Geometry check sheet. Reference: the model listing, model coordinates, mm. A direction names the side the tool comes from. Round coordinates to 2 decimals unless told otherwise and drop trailing zeros. Order: outer loops, then holes, each group sorted by start corner. A loop starts at its lowest first (then second) coordinate and runs counter-clockwise, first axis right, second up.
Autodesk Inventor part; units mm, degrees
ref_plane "YZ Plane" through (0, 0, 0) normal (1, 0, 0) x (0, 1, 0)
ref_plane "XZ Plane" through (0, 0, 0) normal (0, 1, 0) x (-1, 0, 0)
ref_plane "XY Plane" through (0, 0, 0) normal (0, 0, 1) x (1, 0, 0)
sketch "Sketch1" plane through (0, 0, 0) normal (0, 1, 0) x (-1, 0, 0)
  circle A0 centre (0, 0) radius 6
  circle A1 centre (0, 0) radius 22.5
  circle A2 centre (0, 0) radius 9
  line L0 (0, 0) -> (11.3137, -11.3137) construction
  line L1 (0, 0) -> (16, 0) construction
  line L2 (0, 0) -> (-11.3137, 11.3137) construction
  circle A3 centre (11.3137, -11.3137) radius 2.5
  circle A4 centre (-11.3137, 11.3137) radius 2.5
  circle A5 centre (11.3137, 11.3137) radius 2.5
  circle A6 centre (-11.3137, -11.3137) radius 2.5
  dimension "d0" = 12
  dimension "d1" = 45
  dimension "d2" = 18
  dimension "d8" = 45
  dimension "d9" = 16
  dimension "d10" = 5
extrude "Extrusion1" add sketch "Sketch1" along normal blind 20 contours A2
extrude "Extrusion2" add sketch "Sketch1" against normal blind 4 contours A0 | A1 | A2
sketch "Sketch2" plane through (0, 0, 0) normal (1, 0, 0) x (0, 1, 0)
  line L0 (0, 0) -> (10, 0) construction
  circle A0 centre (10, 0) radius 1.5
  dimension "d12" = 10
  dimension "d13" = 3
extrude "Extrusion3" cut sketch "Sketch2" along normal mid plane 30
properties part number "12mm Flange"
(1) Depth check by flat-ended pin: P1, Ø6, axis at x = -3, y = 10.5, coming from the -Z side; P2, Ø5, axis at y = 7, z = -8.5, coming from the -X side; P3, Ø9.5, axis at x = 2, z = -1, coming from the +Y side; P4, Ø4, axis at y = 0.5, z = 17.5, coming from the -X side. Enter the tip coordinate at first touch or a pass-through.
Returned:
P1: stops at z = -9
P2: stops at x = -6.71
P3: stops at y = 20
P4: stops at x = -16.25
(2) Set-up check for faces 1 (the flat face through (-2, 20, -6)), 2 (the flat face through (0, 0, -10)): record each of +Z, -Z, +X, -X, +Y, -Y from which the full face is reachable in a straight line by a thin tool's end or side.
Returned:
face 1: +Z, -Z, +X, -X, +Y
face 2: +Y
(3) Sectioned sample at C-C, the plane y = 10. Record the cut outline in (x, z).
Returned:
outline: (-8.87, -1.5) arc R9 ccw to (8.87, -1.5) - (5.81, -1.5) arc R6 cw to (-5.81, -1.5) - close; (-8.87, 1.5) - (-5.81, 1.5) arc R6 cw to (5.81, 1.5) - (8.87, 1.5) arc R9 ccw to start
(4) Draft check along Z on faces 3 (the cylindrical face through (-13.698, -1.972, -10.563)), 4 (the cylindrical face through (-5.723, 9.86, -1.802)), 5 (the cylindrical face through (-8.584, 9.86, -2.703)), 6 (the flat face through (0, -4, 0)). Enter one of: released by +Z, released by -Z, zero draft, split by the parting line, or undercut.
Returned:
face 3: undercut
face 4: undercut
face 5: split by the parting line
face 6: zero draft
(5) Sectioned sample at A-A, the plane z = 0. Record the cut outline in (x, y).
Returned:
outline: (-22.5, -4) - (22.5, -4) - (22.5, 0) - (9, 0) - (9, 8.5) - (6, 8.5) - (6, 0) - (-6, 0) - (-6, 8.5) - (-9, 8.5) - (-9, 0) - (-22.5, 0) - close; (-9, 11.5) - (-6, 11.5) - (-6, 20) - (-9, 20) - close; (6, 11.5) - (9, 11.5) - (9, 20) - (6, 20) - close
(6) Sectioned sample at B-B, the plane x = 0. Record the cut outline in (y, z).
Returned:
outline: (-4, -22.5) - (0, -22.5) - (0, -9) - (20, -9) - (20, -6) - (0, -6) - (0, 6) - (20, 6) - (20, 9) - (0, 9) - (0, 22.5) - (-4, 22.5) - close
(7) Sectioned sample at D-D, the plane x = -8. Record the cut outline in (y, z).
Returned:
outline: (-4, -21.03) - (0, -21.03) - (0, -4.12) - (20, -4.12) - (20, 4.12) - (0, 4.12) - (0, 21.03) - (-4, 21.03) - close; hole circle Ø3 at (10, 0)
(8) Material ranges on line 1 (Y direction, x = 2.5, z = 9); line 2 (X direction, y = 6.75, z = -0.5); line 3 (X direction, y = 11.5, z = 1), recorded low to high.
Returned:
line 1: y = -4 to 0
line 2: x = -8.99 to -5.98, 5.98 to 8.99
line 3: x = -8.94 to -5.92, 5.92 to 8.94
